Verification items for the finished model (mm, model axes). A direction names the side the tool comes from. Coordinates: 2 decimals unless noted, no trailing zeros. Order: outer loops, then holes, each group sorted by start corner. A loop starts at its lowest first (then second) coordinate and runs counter-clockwise, first axis right, second up. Notation, with made-up numbers: M 35.5,76 L 61.5,76 A26 ccw 61.5,93 Z; hole C 52.25,62.5 d7. An arc over 180 degrees is marked long. Return JSON: item names as keys, results as strings. Group by question number.
1. Set-up check for faces 4 (the flat face through (0, 0, 71.628)), 5 (the flat face through (3, 3, 69.088)): record each of +Z, -Z, +X, -X, +Y, -Y from which the full face is reachable in a straight line by a thin tool's end or side.
2. Section check D-D, the plane z = 30.5. Record the cut outline in (x, y).
3. Section check C-C, the plane z = 9. Record the cut outline in (x, y).
4. Material ranges on line 1 along Y through (x, z) = (0, 9); line 2 along Z through (x, y) = (-2, -1.5); line 3 along Y through (x, z) = (-0.25, 65), recorded low to high.
5. Mould release check, pull along X, two halves, no side actions. Record for faces 1 (the flat face through (1, 3, 0)), 2 (the cylindrical face through (1.699, -3.267, 34.06)), 3 (the cylindrical face through (-0.33, -2.52, 6.26)): +X half, -X half, draft (parallel to the pull), parting line (faces both ways), or undercut.
6. Gauge pin test, flat ends, axial feed: pin 1 (2.5 mm diameter, centred on x = 1, y = -0.5, fed in from -Z); pin 2 (3 mm diameter, centred on y = 0, z = 16.5, fed in from +X); pin 3 (1 mm diameter, centred on x = -1, z = 49.5, fed in from +Y). Record the tip position at first contact, or that the pin passes through.
```python
from build123d import *

# Parameters (mm, degrees)
F0_R     = 3.683
F1_DEPTH = 69.088
F2_R     = 5.08
F3_DEPTH = 2.54
F4_R     = 2.53999
F5_R     = 2.54
F6_DEPTH = 12.7


# Not quite as in the source:
# - a fillet or chamfer is up to 0.001 mm smaller than in the source, because OpenCascade refuses the exact size


with BuildPart() as f1:
    # F0 (on Top) → F1 (new body)
    with BuildSketch(Plane.XY):
        Circle(F0_R)
    extrude(amount=F1_DEPTH)

    # F2 (on face) → F3 (join)
    with BuildSketch(Plane.XY.offset(69.088)):
        Circle(F2_R)
    extrude(amount=F3_DEPTH)

    # F4 (radius 2.54 in the source; OpenCascade refuses exactly that, so slightly less here)
    f4_edges = [f1.edges().sort_by_distance(p)[0] for p in [
        (-5.08, 0, 71.628),
    ]]
    fillet(f4_edges, radius=F4_R)

    # F5 (on face) → F6 (cut)
    with BuildSketch(Plane(origin=(0, 0, 0), x_dir=(1, 0, 0), z_dir=(0, 0, -1))):
        Circle(F5_R)
    extrude(amount=-F6_DEPTH, mode=Mode.SUBTRACT)


solid = f1.part
```
Answers follow:
{
 "1": {"face 4": "+Z, +X, -X, +Y, -Y", "face 5": "-Z"},
 "2": {"outline": "C 0,0 d7.37"},
 "3": {"outline": "C 0,0 d7.37; hole C 0,0 d5.08"},
 "4": {"line 1": "-3.68 to -2.54, 2.54 to 3.68", "line 2": "12.7 to 71.63", "line 3": "-3.67 to 3.67"},
 "5": {"face 1": "draft", "face 2": "parting line", "face 3": "undercut"},
 "6": {"pin 1": "z = 12.7", "pin 2": "x = 3.68", "pin 3": "y = 3.65"}
}
